from build123d import *

# Parameters (mm, degrees)
SM_BASE_FLANGE_1_DEPTH   = 43
SKETCH_6_W               = 14
SKETCH_6_H               = 10
SM_BASE_FLANGE_1_2_DEPTH = 1
SKETCH_9_W               = 3
SKETCH_9_H               = 12
CUT_EXTRUDE_1_DEPTH      = 10
CUT_EXTRUDE_2_DEPTH      = 12
FILLET_1_R               = 1


# Sheet-metal steps are written as plain solids
with BuildPart() as part:
    # Sketch 1 → Sm Base Flange 1 (new body)
    with BuildSketch(Plane(origin=(0, 0, 0), x_dir=(1, 0, 0), z_dir=(0, 1, 0))):
        with BuildLine():
            Line((0, 0), (0, 20))
            ThreePointArc((0, 20), (0.585786438, 21.414213562), (2, 22))
            Line((2, 22), (16, 22))
            ThreePointArc((16, 22), (17.414213562, 21.414213562), (18, 20))
            Line((18, 20), (18, 0))
            Line((18, 0), (17, 0))
            Line((17, 0), (17, 20))
            ThreePointArc((17, 20), (16.707106781, 20.707106781), (16, 21))
            Line((16, 21), (2, 21))
            ThreePointArc((2, 21), (1.292893219, 20.707106781), (1, 20))
            Line((1, 20), (1, 0))
            Line((1, 0), (0, 0))
        make_face()
    extrude(amount=SM_BASE_FLANGE_1_DEPTH)

    # Эскиз6 → Sm Base Flange 1 2 (add)
    with BuildSketch(Plane.ZY):
        with Locations((-7, -5)):
            Rectangle(SKETCH_6_W, SKETCH_6_H)
    extrude(amount=-SM_BASE_FLANGE_1_2_DEPTH)

    # Эскиз9 → Вырез-Вытянуть1 (cut)
    with BuildSketch(Plane(origin=(0, 0, -22), x_dir=(-1, 0, 0), z_dir=(0, 0, -1))):
        with Locations((-6.5, 37)):
            Rectangle(SKETCH_9_W, SKETCH_9_H)
    extrude(amount=-CUT_EXTRUDE_1_DEPTH, mode=Mode.SUBTRACT)

    # Эскиз10 → Вырез-Вытянуть2 (cut)
    with BuildSketch(Plane(origin=(18, 0, 0), x_dir=(0, 0, -1), z_dir=(1, 0, 0))):
        with BuildLine():
            Line((0, 43), (5, 43))
            Line((5, 43), (5, 7))
            ThreePointArc((5, 7), (5.585786438, 5.585786438), (7, 5))
            Line((7, 5), (22, 5))
            Line((22, 5), (22, 0))
            Line((22, 0), (0, 0))
            Line((0, 0), (0, 43))
        make_face()
    extrude(amount=-CUT_EXTRUDE_2_DEPTH, mode=Mode.SUBTRACT)

    # Скругление1
    fillet_1_edges = [part.edges().sort_by_distance(p)[0] for p in [
        (6, 0, -21.5),
        (6, 5, -21.5),
        (0.5, -10, 0),
        (0.5, -10, -14),
        (5, 43, -21.5),
        (5, 31, -21.5),
        (8, 31, -21.5),
        (8, 43, -21.5),
    ]]
    fillet(fillet_1_edges, radius=FILLET_1_R)


solid = part.part
Geometry: final body of the model. Coordinates: model frame, mm. A direction names the side the tool comes from. Round coordinates to 2 decimals unless told otherwise and drop trailing zeros. Loops run counter-clockwise (first coordinate to the right, second up) from the corner with the lowest first, then second, coordinate; pieces in that order, holes last. Notation, with made-up numbers: M 12,-26 L 29,-26 A26 ccw 29,9 Z; hole C 60,62 d2. An arc over 180 degrees is marked long. Put each result on its own line as item: value. Start each with the question number.
(1) Section query A-A (z = -16). Return loops of the section in (x, y).
(2) Contact query for flat-ended pins moving along their axis: pin 1 Ø8 at (x, y) = (7.5, 35.5) entering from +Z; pin 2 Ø1.1 at (x, y) = (0.5, -5) entering from -Z; pin 3 Ø4 at (x, z) = (3.5, -16.5) entering from -Y; pin 4 Ø0.8 at (y, z) = (38.5, -21.5) entering from +X. Output: stop coordinate, or through.
(3) Section query B-B (y = 38). Return loops of the section in (x, z).
(4) Draft query along X for faces 6 (the face through (7.699, 31.285, -21.493)), 7 (the face through (6, 2.5, -21.5)), 8 (the face through (17.4, 5, -16.1)), 9 (the face through (16.715, 23.734, -20.699)). Return one class per face: +X half, -X half, draft (parallel to the pull), parting line (faces both ways), or undercut.
(5) Material intervals for line 1 along X through (y, z) = (19.5, -19.5); line 2 along Z through (x, y) = (4, 10.5); line 3 along X through (y, z) = (-4.5, -3.25), sorted ascending. Write a range as [from, to].
(6) Section query D-D (x = 14.25). Return loops of the section in (y, z).
(7) Set-up query: faces 1 (the face through (1, 17, -10)), 2 (the face through (17.51, 5.6, -5.57)), 3 (the face through (8.285, 42.699, -21.493)), 4 (the face through (17.5, 25.3, -5)), 5 (the face through (0.8, 0, -18.9)). Return all of +Z, -Z, +X, -X, +Y, -Y with unobstructed straight access to the full face (end or side cutting, diameter ignored); none if empty.
(8) Section query C-C (z = -9). Return loops of the section in (x, y), then the cut area to 3 significant figures.
Findings below:
1. outline: M 0,0 L 1,0 L 1,43 L 0,43 Z; M 17,5 L 18,5 L 18,43 L 17,43 Z
2. pin 1: stops at z = -21
2. pin 2: stops at z = -14
2. pin 3: passes through
2. pin 4: stops at x = 17.67
3. outline: M 0,-20 A2 ccw 2,-22 L 5,-22 L 5,-21 L 2,-21 A1 cw 1,-20 L 1,0 L 0,0 Z; M 8,-22 L 16,-22 A2 ccw 18,-20 L 18,-5 L 17,-5 L 17,-20 A1 cw 16,-21 L 8,-21 Z
4. face 6: undercut
4. face 7: +X half
4. face 8: draft
4. face 9: undercut
5. line 1: x = [0, 1], [17, 18]
5. line 2: z = [-22, -21]
5. line 3: x = [0, 1]
6. outline: M 5,-22 L 43,-22 L 43,-21 L 5,-21 Z
7. face 1: +Z, +Y, -Y
7. face 2: +Z, +X, -Y
7. face 3: +Z, -Z, +Y
7. face 4: +Z, +X, +Y, -Y
7. face 5: -Z, +X, -X, -Y
8. outline: M 0,-10 L 1,-10 L 1,43 L 0,43 Z; M 17,5 L 18,5 L 18,43 L 17,43 Z
8. area: 91.0 mm2
